The model under review builds one solid part; all positions refer to its coordinate system, in mm. A direction names the side the tool comes from. Coordinates: 2 decimals unless noted, no trailing zeros. Loops run counter-clockwise (first coordinate to the right, second up) from the corner with the lowest first, then second, coordinate; pieces in that order, holes last. Notation, with made-up numbers: (57.5, 51) - (107.5, 51) arc R30 cw to (107.5, 79) - close; hole circle Ø9 at (16, 11). An arc over 180 degrees is marked (long way). Answer in a Markdown table with one row per item. Add a question column.
(1) We need section D-D on z = -7.5. Write out the cut boundary in (x, y).
(2) Mouldability with a two-part tool opening along X and no side actions: class faces 6 (the flat face through (6, 7, -24)), 7 (the cylindrical face through (0, 2, -40)), 8 (the flat face through (24.3, 7.5, 7.1)) as +X half, -X half, draft (parallel to the pull), parting line (faces both ways), or undercut.
(3) We need section C-C on x = -12.5. Write out the cut boundary in (y, z), plus the area to 3 significant figures.
(4) We need section B-B on z = -22. Write out the cut boundary in (x, y), plus the area to 3 significant figures.
(5) For line 1 along Z through (x, y) = (24.5, 4.5); line 2 along X through (y, z) = (9.5, -20.5); line 3 along Z through (x, y) = (-27, 3.5), list the stretches that pass through material, from the lowest coordinate up.
(6) For P1, Ø5.5, axis at y = 6.5, z = 26, coming from the +X side; P2, Ø6.5, axis at x = 0, z = -30, coming from the -Y side; P3, Ø2, axis at x = 6, y = 2, coming from the -Z side; P4, Ø2.5, axis at y = 3, z = -20.5, coming from the -X side, all flat-tipped, find the tip position at first contact; note any pin that passes through.
(7) Machinability: for faces 1 (the flat face through (15.414, 2.465, 20.446)), 2 (the flat face through (15.567, 2.465, -20.535)), 3 (the flat face through (-32, 5, -13)), 4 (the flat face through (18.19, 7.46, 17.43)), 5 (the cylindrical face through (9.95, 7.46, -17.35)), which of the approach directions +Z, -Z, +X, -X, +Y, -Y give a long, thin tool a straight path to every point of the face, cutting with its end or side? Answer none if there is none.
(8) We need section A-A on x = 0. Write out the cut boundary in (y, z).
Autodesk Fusion 360 part; units mm, degrees
sketch "Sketch1" plane through (0, 0, 0) normal (0, 1, 0) x (1, 0, 0)
  circle A0 centre (0, 0) radius 16
  circle A1 centre (0, 0) radius 30 construction
  arc A2 (-6, -30) -> (6, -30) centre (0, -30) ccw
  arc A3 (6, 30) -> (-6, 30) centre (0, 30) ccw
  arc A4 (-10, -30) -> (10, -30) centre (0, -30) ccw
  arc A5 (10, 30) -> (-10, 30) centre (0, 30) ccw
  circle A6 centre (0, 0) radius 20
  line L0 (-10, 30) -> (-10, 17.3205)
  line L1 (-10, -17.3205) -> (-10, -30)
  line L2 (-6, 30) -> (-6, 19.0788)
  line L3 (-6, -19.0788) -> (-6, -30)
  line L4 (0, 30) -> (0, 20) construction
  line L5 (0, -16) -> (0, -30) construction
  line L6 (6, -30) -> (6, -19.0788)
  line L7 (6, 19.0788) -> (6, 30)
  line L8 (10, -30) -> (10, -17.3205)
  line L9 (10, 17.3205) -> (10, 30)
  line L10 (-20, 0) -> (-30.9808, -6.3397)
  line L11 (-19.5227, -4.3432) -> (-28.9808, -9.8038)
  line L12 (-22.9808, -20.1962) -> (-13.5227, -14.7355)
  line L13 (-20.9808, -23.6603) -> (-10, -17.3205)
  arc A7 (-30.9808, -6.3397) -> (-20.9808, -23.6603) centre (-25.9808, -15) ccw
  arc A8 (-28.9808, -9.8038) -> (-22.9808, -20.1962) centre (-25.9808, -15) ccw
  line L14 (20, 0) -> (30.9808, 6.3397)
  line L15 (19.5227, 4.3432) -> (28.9808, 9.8038)
  line L16 (22.9808, 20.1962) -> (13.5227, 14.7355)
  line L17 (20.9808, 23.6603) -> (10, 17.3205)
  arc A9 (30.9808, 6.3397) -> (20.9808, 23.6603) centre (25.9808, 15) ccw
  arc A10 (28.9808, 9.8038) -> (22.9808, 20.1962) centre (25.9808, 15) ccw
  line L18 (10, -17.3205) -> (20.9808, -23.6603)
  line L19 (13.5227, -14.7355) -> (22.9808, -20.1962)
  line L20 (28.9808, -9.8038) -> (19.5227, -4.3432)
  line L21 (30.9808, -6.3397) -> (20, 0)
  arc A11 (20.9808, -23.6603) -> (30.9808, -6.3397) centre (25.9808, -15) ccw
  arc A12 (22.9808, -20.1962) -> (28.9808, -9.8038) centre (25.9808, -15) ccw
  line L22 (-10, 17.3205) -> (-20.9808, 23.6603)
  line L23 (-13.5227, 14.7355) -> (-22.9808, 20.1962)
  line L24 (-28.9808, 9.8038) -> (-19.5227, 4.3432)
  line L25 (-30.9808, 6.3397) -> (-20, 0)
  arc A13 (-20.9808, 23.6603) -> (-30.9808, 6.3397) centre (-25.9808, 15) ccw
  arc A14 (-22.9808, 20.1962) -> (-28.9808, 9.8038) centre (-25.9808, 15) ccw
  dimension "d1" = 32
  dimension "d2" = 60
  dimension "d3" = 12
  dimension "d5" = 40
  dimension "d7" = 360
extrude "Extrude1" add sketch "Sketch1" along normal blind 10 contours A2 A6 L3 L6 | A6 | A6 L11 L12 A8 | A6 L19 L20 A12 | A6 L23 L24 A14 | A6 L15 L16 A10 | A3 A6 L2 L7
extrude "Extrude2" add sketch "Sketch1" along normal blind 5 contours A2 A4 A6 L1 L3 L6 L8 | A6 L10 L11 L12 L13 A7 A8 | A6 L18 L19 L20 L21 A11 A12 | A6 L22 L23 L24 L25 A13 A14 | A6 L14 L15 L16 L17 A9 A10 | A3 A5 A6 L0 L2 L7 L9
hole "Hole1" at (0, 0, -30) direction (0, 1, 0) diameter 8 end through all
pattern_circular "C-Pattern1" count 6 over 360 about axis through (0, 1.75, 0) along (0, 1, 0) of "Hole1"
Outcome:
| question | item | result |
|---|---|---|
| 1 | outline | (-32.6, 0) - (-14.13, 0) - (-14.13, 10) - (-24.99, 10) - (-24.99, 5) - (-32.6, 5) - close; (14.13, 0) - (32.6, 0) - (32.6, 5) - (24.99, 5) - (24.99, 10) - (14.13, 10) - close |
| 2 | face 6 | undercut |
| 2 | face 7 | parting line |
| 2 | face 8 | +X half |
| 3 | outline | (0, -18.76) - (5, -18.76) - (5, -15.61) - (10, -15.61) - (10, -9.99) - (0, -9.99) - close; (0, 9.99) - (10, 9.99) - (10, 15.61) - (5, 15.61) - (5, 18.76) - (0, 18.76) - close |
| 3 | area | 144 mm² |
| 4 | outline | (-33.12, 0) - (-18.11, 0) - (-18.11, 5) - (-33.12, 5) - close; (-10, 0) - (10, 0) - (10, 5) - (6, 5) - (6, 10) - (-6, 10) - (-6, 5) - (-10, 5) - close; (18.11, 0) - (33.12, 0) - (33.12, 5) - (18.11, 5) - close |
| 4 | area | 310 mm² |
| 5 | line 1 | -24.89 to -18.72, -11.28 to -2.6, 2.6 to 11.28, 18.72 to 24.89 |
| 5 | line 2 | -28.38 to -23.58, -6 to 6, 23.58 to 28.38 |
| 5 | line 3 | -24.95 to -18.87, -11.13 to -4.04, 4.04 to 11.13, 18.87 to 24.95 |
| 6 | P1 | x = 30.92 |
| 6 | P2 | through |
| 6 | P3 | z = -38.66 |
| 6 | P4 | x = -35.03 |
| 7 | face 1 | +Z, +Y, -Y |
| 7 | face 2 | -Z, +Y, -Y |
| 7 | face 3 | +Y |
| 7 | face 4 | +Z, +Y |
| 7 | face 5 | -Z, +Y |
| 8 | outline | (0, -40) - (5, -40) - (5, -36) - (10, -36) - (10, -34) - (0, -34) - close; (0, -26) - (10, -26) - (10, -16) - (0, -16) - close; (0, 16) - (10, 16) - (10, 26) - (0, 26) - close; (0, 34) - (10, 34) - (10, 36) - (5, 36) - (5, 40) - (0, 40) - close |
